from build123d import *

# Parameters (mm, degrees)
BOSS_EXTRUDE1_DEPTH = 6.35
SKETCH2_R           = 1.5
CUT_EXTRUDE1_DEPTH  = 7.35
SKETCH3_R           = 1.25
CUT_EXTRUDE2_DEPTH  = 7.35


with BuildPart() as part:
    # Sketch1 → Boss-Extrude1 (new body)
    with BuildSketch(Plane(origin=(0, 0, 0), x_dir=(1, 0, 0), z_dir=(0, 1, 0))):
        Polygon((50.8, 121.285), (76.2, 121.285), (76.2, 19.05), (82.55, 19.05), (82.55, 6.35), (76.2, 6.35), (76.2, 0), (0, 0), (0, 6.35), (-6.35, 6.35), (-6.35, 19.05), (0, 19.05), (0, 121.285), (25.4, 121.285), (25.4, 127.635), (50.8, 127.635), align=None)
    extrude(amount=BOSS_EXTRUDE1_DEPTH)

    # Sketch2 → Cut-Extrude1 (cut, through all)
    with BuildSketch(Plane(origin=(0, 6.35, 0), x_dir=(1, 0, 0), z_dir=(0, 1, 0))):
        with Locations((35.0139, 6.096)):
            Circle(SKETCH2_R)
    extrude(amount=-CUT_EXTRUDE1_DEPTH, mode=Mode.SUBTRACT)

    # Sketch3 → Cut-Extrude2 (cut, through all)
    with BuildSketch(Plane(origin=(0, 6.35, 0), x_dir=(1, 0, 0), z_dir=(0, 1, 0))):
        with Locations((-3.175, 12.7)):
            Circle(SKETCH3_R)
        with Locations((79.375, 12.7)):
            Circle(SKETCH3_R)
        with Locations((38.1, 124.46)):
            Circle(SKETCH3_R)
    extrude(amount=-CUT_EXTRUDE2_DEPTH, mode=Mode.SUBTRACT)


solid = part.part
Model file for the job. Use its own axes, mm. A direction names the side the tool comes from. Round coordinates to 2 decimals unless told otherwise and drop trailing zeros. Order: outer loops, then holes, each group sorted by start corner. A loop starts at its lowest first (then second) coordinate and runs counter-clockwise, first axis right, second up.
(1) Band-saw the part on A-A (z = -12.7). List the corners of the cut face in (x, y) (3 decimals), then the cut area to 3 significant figures.
(2) 3-axis set-ups, long thin cutter, end or side, ignore diameter. For faces 5 (the face through (0, 3, -69)), 6 (the face through (39, 6.35, -65)), 7 (the face through (-3.34, 3.22, -13.94)), 8 (the face through (-3, 3, -6.35)), 9 (the face through (63, 3, -121.285)): which of +Z, -Z, +X, -X, +Y, -Y reach the whole face in a straight line?
(3) Drill centre lines: line 1 (X direction, y = 3, z = -12.7) (3 decimals); line 2 (Z direction, x = 38.1, y = 2.5) (3 decimals); line 3 (X direction, y = 3, z = -124.46). Where is each one in solid material? Low to high.
(4) Pull direction X, two halves, no side cores. Call faces 1 (the face through (80.567, 3.219, -13.075)), 2 (the face through (79, 3, -6.35)), 3 (the face through (0, 3, -3)), 4 (the face through (76.2, 3, -3)): released by +X, released by -X, zero draft, split by the parting line, or undercut.
(5) Band-saw the part on B-B (x = 38.1). List the corners of the cut face in (y, z) (3 decimals).
(6) Band-saw the part on C-C (z = -124.46). List the corners of the cut face in (x, y).
(7) Pin check, flat tips, straight feed: pin 1 (3 mm diameter, centred on y = 3.5, z = -125, fed in from +X); pin 2 (3 mm diameter, centred on x = 79.5, y = 4, fed in from +Z); pin 3 (1 mm diameter, centred on y = 5.5, z = -88, fed in from +X); pin 4 (2 mm diameter, centred on x = 79.375, z = -12.7, fed in from +Y). Stop position of each tip, or through.
(8) Band-saw the part on D-D (y = 4.25). List the corners of the cut face in (x, z) (3 decimals), then the cut area to 3 significant figures.
Verdict:
1. outline: (-6.35, 0) - (-4.425, 0) - (-4.425, 6.35) - (-6.35, 6.35) - close; (-1.925, 0) - (78.125, 0) - (78.125, 6.35) - (-1.925, 6.35) - close; (80.625, 0) - (82.55, 0) - (82.55, 6.35) - (80.625, 6.35) - close
1. area: 533 mm2
2. face 5: -Z, -X, +Y, -Y
2. face 6: +Z, -Z, +X, -X, +Y
2. face 7: +Y, -Y
2. face 8: +Z, -X, +Y, -Y
2. face 9: -Z, +X, +Y, -Y
3. line 1: x = -6.35 to -4.425, -1.925 to 78.125, 80.625 to 82.55
3. line 2: z = -127.635 to -125.71, -123.21 to 0
3. line 3: x = 25.4 to 36.85, 39.35 to 50.8
4. face 1: undercut
4. face 2: zero draft
4. face 3: released by -X
4. face 4: released by +X
5. outline: (0, -127.635) - (6.35, -127.635) - (6.35, -125.71) - (0, -125.71) - close; (0, -123.21) - (6.35, -123.21) - (6.35, 0) - (0, 0) - close
6. outline: (25.4, 0) - (36.85, 0) - (36.85, 6.35) - (25.4, 6.35) - close; (39.35, 0) - (50.8, 0) - (50.8, 6.35) - (39.35, 6.35) - close
7. pin 1: stops at x = 50.8
7. pin 2: stops at z = -6.35
7. pin 3: stops at x = 76.2
7. pin 4: passes through
8. outline: (-6.35, -19.05) - (0, -19.05) - (0, -121.285) - (25.4, -121.285) - (25.4, -127.635) - (50.8, -127.635) - (50.8, -121.285) - (76.2, -121.285) - (76.2, -19.05) - (82.55, -19.05) - (82.55, -6.35) - (76.2, -6.35) - (76.2, 0) - (0, 0) - (0, -6.35) - (-6.35, -6.35) - close; hole circle Ø2.5 at (-3.175, -12.7); hole circle Ø3 at (35.014, -6.096); hole circle Ø2.5 at (38.1, -124.46); hole circle Ø2.5 at (79.375, -12.7)
8. area: 9,540 mm2
